Read the model definition and answer for the solid it produces. Units are mm, in the model's axes. A direction names the side the tool comes from. Round coordinates to 2 decimals unless told otherwise and drop trailing zeros. Order: outer loops, then holes, each group sorted by start corner. A loop starts at its lowest first (then second) coordinate and runs counter-clockwise, first axis right, second up.
from build123d import *

# Parameters (mm, degrees)
SKETCH030_R     = 3.9
PAD005_DEPTH    = 1.8
SKETCH029_R     = 2.6
PAD006_DEPTH    = 11.5
SKETCH033_R     = 2.6
POCKET_DEPTH    = 14
POCKET011_DEPTH = 5
SKETCH034_R     = 3.15
POCKET012_DEPTH = 7.8
POCKET013_DEPTH = 16
SKETCH036_R     = 2
POCKET014_DEPTH = 16
SKETCH037_R     = 4.2
POCKET015_DEPTH = 13


with BuildPart() as part:
    # Sketch → Revolution (revolve)
    with BuildSketch(Plane.XZ):
        Polygon((13.5, 21), (13.5, 23.5), (14.3, 23.5), (14.8, 23), (14.8, 16.5), (16.75, 16.5), (16.75, 16), (30, 16), (30, 11.5), (40, 11.5), (40, 0), (10, 0), (9, 1), (9, 20.5), (9.5, 21), align=None)
    revolve(axis=Axis((0, 0, 0), (0, 0, 1)))

    # Sketch030 → Pad005 (new body)
    with BuildSketch(Plane.XY.offset(11.5)):
        with Locations((-25, -35)):
            Circle(SKETCH030_R)
        with Locations((25, -35)):
            Circle(SKETCH030_R)
    extrude(amount=PAD005_DEPTH)

    # Sketch029 → Pad006 (join)
    with BuildSketch(Plane.XY):
        with BuildLine():
            Line((-30, -26.457513), (-30, -43.542487))
            ThreePointArc((-30, -43.542487), (0, -110), (30, -43.542487))
            Line((30, -26.457513), (30, -43.542487))
            ThreePointArc((-30, -26.457513), (0, -40), (30, -26.457513))
        make_face()
        with Locations((0, -70)):
            Circle(SKETCH029_R, mode=Mode.SUBTRACT)
    extrude(amount=PAD006_DEPTH)

    # Sketch033 → Pocket (cut)
    with BuildSketch(Plane.XY):
        with Locations((-25, -35)):
            Circle(SKETCH033_R)
        with Locations((25, -35)):
            Circle(SKETCH033_R)
    extrude(amount=POCKET_DEPTH, mode=Mode.SUBTRACT)

    # Sketch031 → Pocket011 (cut)
    with BuildSketch(Plane.XY.offset(6.5)):
        with BuildLine():
            ThreePointArc((27.091167, -29.564821), (0, 40.1), (-27.091167, -29.564821))
            Line((-25.672428, -28.016539), (-27.091167, -29.564821))
            ThreePointArc((25.672428, -28.016539), (0, 38), (-25.672428, -28.016539))
            Line((25.672428, -28.016539), (27.091167, -29.564821))
        make_face()
        with BuildLine():
            ThreePointArc((-27.091167, -40.435179), (0, -110.1), (27.091167, -40.435179))
            Line((27.091167, -40.435179), (25.672428, -41.983461))
            ThreePointArc((-25.672428, -41.983461), (0, -108), (25.672428, -41.983461))
            Line((-27.091167, -40.435179), (-25.672428, -41.983461))
        make_face()
    extrude(amount=POCKET011_DEPTH, mode=Mode.SUBTRACT)

    # Sketch034 → Pocket012 (cut)
    with BuildSketch(Plane.XY):
        with Locations((-25, -35)):
            Circle(SKETCH034_R)
        with Locations((25, -35)):
            Circle(SKETCH034_R)
    extrude(amount=POCKET012_DEPTH, mode=Mode.SUBTRACT)

    # Sketch035 → Pocket013 (cut)
    with BuildSketch(Plane.XY):
        with BuildLine():
            Line((-6, -7), (-6, -20))
            ThreePointArc((-6, -20), (0, -26), (6, -20))
            Line((6, -7), (6, -20))
            Line((-6, -7), (6, -7))
        make_face()
    extrude(amount=POCKET013_DEPTH, mode=Mode.SUBTRACT)

    # Sketch036 → Pocket014 (cut)
    with BuildSketch(Plane.XY):
        with Locations((-19, -6)):
            Circle(SKETCH036_R)
        with Locations((19, -6)):
            Circle(SKETCH036_R)
    extrude(amount=POCKET014_DEPTH, mode=Mode.SUBTRACT)

    # Sketch037 → Pocket015 (cut)
    with BuildSketch(Plane.XY.offset(4)):
        with Locations((-19, -6)):
            Circle(SKETCH037_R)
        with Locations((19, -6)):
            Circle(SKETCH037_R)
    extrude(amount=POCKET015_DEPTH, mode=Mode.SUBTRACT)


solid = part.part
Q1. A cutting plane is placed at D-D, the plane y = -70. Give the vertices of the cut face in (x, z), plus the area to 3 significant figures.
Outcome:
outline: (-40, 0) - (-2.6, 0) - (-2.6, 11.5) - (-38, 11.5) - (-38, 6.5) - (-40, 6.5) - close; (2.6, 0) - (40, 0) - (40, 6.5) - (38, 6.5) - (38, 11.5) - (2.6, 11.5) - close
area: 840 mm2
Q2. For a pull along X with two mould halves and no side action, classify faces 1 (the face through (-24, -38, 13.3)), 2 (the face through (-20.6, -7.2, 2)), 3 (the face through (-6, -13, 8)), 4 (the face through (-3.208, -14.448, 19.704)) as released by +X, released by -X, zero draft, split by the parting line, or undercut.
Outcome:
face 1: zero draft
face 2: undercut
face 3: undercut
face 4: split by the parting line
Q3. A cutting plane is placed at C-C, the plane x = 0. Give the number of separate pieces and of enclosed holes in the cut face, plus the area to 3 significant figures.
Outcome:
separate pieces: 4
enclosed holes: 0
area: 1,420 mm2
Q4. For faces 5 (the face through (-0.261, -16.748, 16.247)), 6 (the face through (-30, -35, 6)), 7 (the face through (-17, -7, 4)), determine the directions among +Z, -Z, +X, -X, +Y, -Y from which every point of the face is accessible in a straight line to the end or side of a thin tool.
Outcome:
face 5: +Z, -Y
face 6: +Z, -Z, -X
face 7: +Z
Q5. Straight lines are drawn through the part: probe 1 along X at (y, z) = (-6, 8.5); probe 2 along Y at (x, z) = (21.5, 12.25); probe 3 along Z at (x, y) = (31.5, -56). For each, find the intervals that lie inside material, in ascending order.
Outcome:
probe 1: x = -37.52 to -23.2, -14.8 to -6.71, 6.71 to 14.8, 23.2 to 37.52
probe 2: y = -36.72 to -33.28, -20.92 to -9.37, -2.63 to 20.92
probe 3: z = 0 to 11.5
Q6. Flat-ended cylindrical pins translate along their axes: pin 1 (6.5 mm diameter, centred on x = -20.5, y = -7.5, fed in from +Z); pin 2 (4 mm diameter, centred on x = -4.5, z = 7, fed in from -Y); pin 3 (5 mm diameter, centred on x = 30.5, z = 8.5, fed in from +Y). Find the tip coordinate at first contact, or state that the pin passes through.
Outcome:
pin 1: stops at z = 16
pin 2: stops at y = -109.92
pin 3: stops at y = 27.55
Q7. A cutting plane is placed at B-B, the plane x = 35. Give the vertices of the cut face in (y, z).
Outcome:
outline: (-89.36, 0) - (-50.64, 0) - (-50.64, 6.5) - (-55.2, 6.5) - (-55.2, 11.5) - (-84.8, 11.5) - (-84.8, 6.5) - (-89.36, 6.5) - close; (-19.36, 0) - (19.36, 0) - (19.36, 6.5) - (14.8, 6.5) - (14.8, 11.5) - (-14.8, 11.5) - (-14.8, 6.5) - (-19.36, 6.5) - close
